from build123d import *

# Parameters (mm, degrees)
SKETCH1_W           = 125
SKETCH1_H           = 18
BOSS_EXTRUDE1_DEPTH = 5
SKETCH3_W           = 125
SKETCH3_H           = 5
BOSS_EXTRUDE2_DEPTH = 15
SKETCH5_R           = 2
CUT_EXTRUDE1_DEPTH  = 6
SKETCH6_R           = 1.75
CUT_EXTRUDE2_DEPTH  = 6


with BuildPart() as part:
    # Sketch1 → Boss-Extrude1 (new body)
    with BuildSketch(Plane(origin=(0, 0, 0), x_dir=(1, 0, 0), z_dir=(0, 1, 0))):
        with Locations((62.5, 9)):
            Rectangle(SKETCH1_W, SKETCH1_H)
    extrude(amount=-BOSS_EXTRUDE1_DEPTH)

    # Sketch3 → Boss-Extrude2 (add)
    with BuildSketch(Plane(origin=(0, 0, 0), x_dir=(1, 0, 0), z_dir=(0, 1, 0))):
        with Locations((62.5, 15.5)):
            Rectangle(SKETCH3_W, SKETCH3_H)
    extrude(amount=BOSS_EXTRUDE2_DEPTH)

    # Sketch5 → Cut-Extrude1 (cut, through all)
    with BuildSketch(Plane.XY.offset(-13)):
        with Locations((25, 7.5)):
            Circle(SKETCH5_R)
        with Locations((100, 7.5)):
            Circle(SKETCH5_R)
    extrude(amount=-CUT_EXTRUDE1_DEPTH, mode=Mode.SUBTRACT)

    # Sketch6 → Cut-Extrude2 (cut, through all)
    with BuildSketch(Plane(origin=(0, 0, 0), x_dir=(1, 0, 0), z_dir=(0, 1, 0))):
        with Locations((35, 6.5)):
            Circle(SKETCH6_R)
        with Locations((90, 6.5)):
            Circle(SKETCH6_R)
    extrude(amount=-CUT_EXTRUDE2_DEPTH, mode=Mode.SUBTRACT)


solid = part.part
Verification items for the finished model (mm, model axes). A direction names the side the tool comes from. Give positions to 0.01 mm unless a question says otherwise; leave off trailing zeros. Order: outer loops, then holes, each group sorted by start corner. A loop starts at its lowest first (then second) coordinate and runs counter-clockwise, first axis right, second up. Notation, with made-up numbers: M 41.5,44.5 L 85.5,44.5 A7 cw 85.5,57.5 Z; hole C -35,40 d9. An arc over 180 degrees is marked long. Answer as a JSON object with one key per item and string values. Group by question number.
1) Access from +Z, -Z, +X, -X, +Y, -Y to the whole of each face (thin tool, end or side, straight path). Record for faces 1 (the face through (62, 15, -16)), 2 (the face through (62, 7, -13)).
2) Mould release check, pull along X, two halves, no side actions. Record for faces 3 (the face through (0, 0, -15)), 4 (the face through (23.526, 8.852, -15.465)), 5 (the face through (89.62, -2.46, -4.79)), 6 (the face through (62, 0, -7)): released by +X, released by -X, zero draft, split by the parting line, or undercut.
3) Cross-section at A-A (x = 100). Enter the section's corners in (y, z).
4) Cross-section at B-B (z = -6.5). Enter the section's corners in (x, y), then the cut area to 3 significant figures.
5) Scan lines: line 1 along X through (y, z) = (-1.2, -6.5); line 2 along Y through (x, z) = (100, -16.3); line 3 along Z through (x, y) = (90, -1.85). Record each from-to range of solid material in increasing order. Write a range as [from, to].
6) Cross-section at C-C (x = 57). Enter the section's corners in (y, z), then the cut area to 3 significant figures.
7) Depth check by flat-ended pin: pin 1 Ø5 at (y, z) = (3, -8.5) entering from +X; pin 2 Ø4.5 at (x, y) = (40.5, 8.5) entering from +Z; pin 3 Ø6.5 at (x, z) = (58.5, -5) entering from +Y. Enter the tip coordinate at first touch or a pass-through.
8) Cross-section at D-D (y = 1.75). Enter the section's corners in (x, z), then the cut area to 3 significant figures.
Result sheet:
{
 "1": {"face 1": "+Z, -Z, +X, -X, +Y", "face 2": "+Z, +X, -X, +Y"},
 "2": {"face 3": "released by -X", "face 4": "undercut", "face 5": "undercut", "face 6": "zero draft"},
 "3": {"outline": "M -5,-18 L 5.5,-18 L 5.5,-13 L 0,-13 L 0,0 L -5,0 Z; M 9.5,-18 L 15,-18 L 15,-13 L 9.5,-13 Z"},
 "4": {"outline": "M 0,-5 L 33.25,-5 L 33.25,0 L 0,0 Z; M 36.75,-5 L 88.25,-5 L 88.25,0 L 36.75,0 Z; M 91.75,-5 L 125,-5 L 125,0 L 91.75,0 Z", "area": "590 mm2"},
 "5": {"line 1": "x = [0, 33.25], [36.75, 88.25], [91.75, 125]", "line 2": "y = [-5, 5.5], [9.5, 15]", "line 3": "z = [-18, -8.25], [-4.75, 0]"},
 "6": {"outline": "M -5,-18 L 15,-18 L 15,-13 L 0,-13 L 0,0 L -5,0 Z", "area": "165 mm2"},
 "7": {"pin 1": "passes through", "pin 2": "stops at z = -13", "pin 3": "stops at y = 0"},
 "8": {"outline": "M 0,-18 L 125,-18 L 125,-13 L 0,-13 Z", "area": "625 mm2"}
}
